Design review of the part built by this model. Coordinates are the model's own, in mm. A direction names the side the tool comes from. Round coordinates to 2 decimals unless told otherwise and drop trailing zeros. Loops run counter-clockwise (first coordinate to the right, second up) from the corner with the lowest first, then second, coordinate; pieces in that order, holes last. Notation, with made-up numbers: (-1.75, 21) - (39.25, 21) arc R10 cw to (39.25, 28) - close; hole circle Ø7 at (85.25, 33.5). An arc over 180 degrees is marked (long way). Answer as CSV lines item,"result". Start each with the question number.
(1) Consider section C-C (z = -8.25). Give the boundary of the cut face in (x, y), and give its area (3 significant figures).
(2) Consider section A-A (y = 2.95). Give the boundary of the cut face in (x, z), and give its area (3 significant figures).
(3) For P1, Ø5, axis at x = -10, z = -11, coming from the -Y side; P2, Ø1.8, axis at x = -13.5, z = -4, coming from the +Y side; P3, Ø2, axis at y = 4, z = -2.5, coming from the -X side, all flat-tipped, find the tip position at first contact; note any pin that passes through.
(4) For faces 1 (the flat face through (-8, 3, -13.6)), 2 (the flat face through (-13, 2.6, -7)), list the 3-axis set-ups (+Z, -Z, +X, -X, +Y, -Y) from which the entire face can be reached by the end or side of a thin tool; tool diameter is ignored.
(5) Consider section B-B (z = -3.75). Give the boundary of the cut face in (x, y), and give its area (3 significant figures).
(6) Mouldability with a two-part tool opening along X and no side actions: class faces 3 (the flat face through (-6, 5.2, -7)), 4 (the flat face through (-11.7, 4, -7)), 5 (the cylindrical face through (-9.595, 3.141, -1.003)) as released by +X, released by -X, zero draft, split by the parting line, or undercut.
(7) Wall thickness on L1, parallel to Z at x = -9.7, y = 3.95; L2, parallel to X at y = 3.95, z = -11; L3, parallel to Z at x = -8.5, y = 2.4: over which ranges is each line inside the solid? List them lowest first.
Autodesk Inventor part; units mm, degrees
ref_plane "YZ Plane" through (0, 0, 0) normal (1, 0, 0) x (0, 1, 0)
ref_plane "XZ Plane" through (0, 0, 0) normal (0, 1, 0) x (-1, 0, 0)
ref_plane "XY Plane" through (0, 0, 0) normal (0, 0, 1) x (1, 0, 0)
sketch "Sketch1" plane through (0, 0, 0) normal (0, 1, 0) x (-1, 0, 0)
  line L0 (0, 0) -> (15.2, 0)
  line L1 (15.2, 0) -> (15.2, -13.6)
  line L2 (15.2, -13.6) -> (0, -13.6)
  line L3 (0, -13.6) -> (0, 0)
  circle A0 centre (9.7, -2.6) radius 1.6
  circle A1 centre (9.7, -11) radius 1.6
  line L4 (9.7, 0) -> (9.7, -13.6) construction
  dimension "d0" = 13.6
  dimension "d1" = 15.2
  dimension "d2" = 3.2
  dimension "d3" = 2.6
  dimension "d4" = 2.6
  dimension "d5" = 5.5
extrude "Extrusion1" add sketch "Sketch1" along normal blind 2.6
sketch "Sketch2" plane through (0, 2.6, 0) normal (0, 1, 0) x (1, 0, 0)
  line L0 (0, 0) -> (0, 13.6)
  line L1 (0, 13.6) -> (-15.2, 13.6)
  line L2 (0, 0) -> (-11.7, 0)
  line L3 (-11.7, 0) -> (-11.7, 13.6)
  line L4 (-11.7, 13.6) -> (0, 13.6)
  line L5 (0, 13.6) -> (0, 0)
  line L6 (-15.2, 13.6) -> (-15.2, 0)
  circle A0 centre (-9.7, 11) radius 1.6
  circle A1 centre (-9.7, 2.6) radius 1.6
  circle A2 centre (-9.7, 2.6) radius 1.6
  circle A3 centre (-9.7, 11) radius 1.6
  point P0 (-15.2, 6.8)
  dimension "d9" = 3.5
extrude "Extrusion3" add sketch "Sketch2" along normal blind 2.6
properties part number "micro usb pin cover"
Determined:
1,outline,"(-15.2, 0) - (0, 0) - (0, 5.2) - (-11.7, 5.2) - (-11.7, 2.6) - (-15.2, 2.6) - close"
1,area,"69.9 mm^2"
2,outline,"(-11.7, -13.6) - (0, -13.6) - (0, 0) - (-11.7, 0) - close; hole circle Ø3.2 at (-9.7, -11); hole circle Ø3.2 at (-9.7, -2.6)"
2,area,"143 mm^2"
3,P1,"stops at y = 0"
3,P2,"stops at y = 2.6"
3,P3,"stops at x = -11.7"
4,face 1,"-Z, +X, -X, +Y, -Y"
4,face 2,"+Z, -Z, -X, +Y"
5,outline,"(-15.2, 0) - (-10.81, 0) - (-10.81, 5.2) - (-11.7, 5.2) - (-11.7, 2.6) - (-15.2, 2.6) - close; (-8.59, 0) - (0, 0) - (0, 5.2) - (-8.59, 5.2) - close"
5,area,"58.4 mm^2"
6,face 3,"zero draft"
6,face 4,"released by -X"
6,face 5,"undercut"
7,L1,"z = -13.6 to -12.6, -9.4 to -4.2, -1 to 0"
7,L2,"x = -11.7 to -11.3, -8.1 to 0"
7,L3,"z = -13.6 to -12.06, -9.94 to -3.66, -1.54 to 0"
